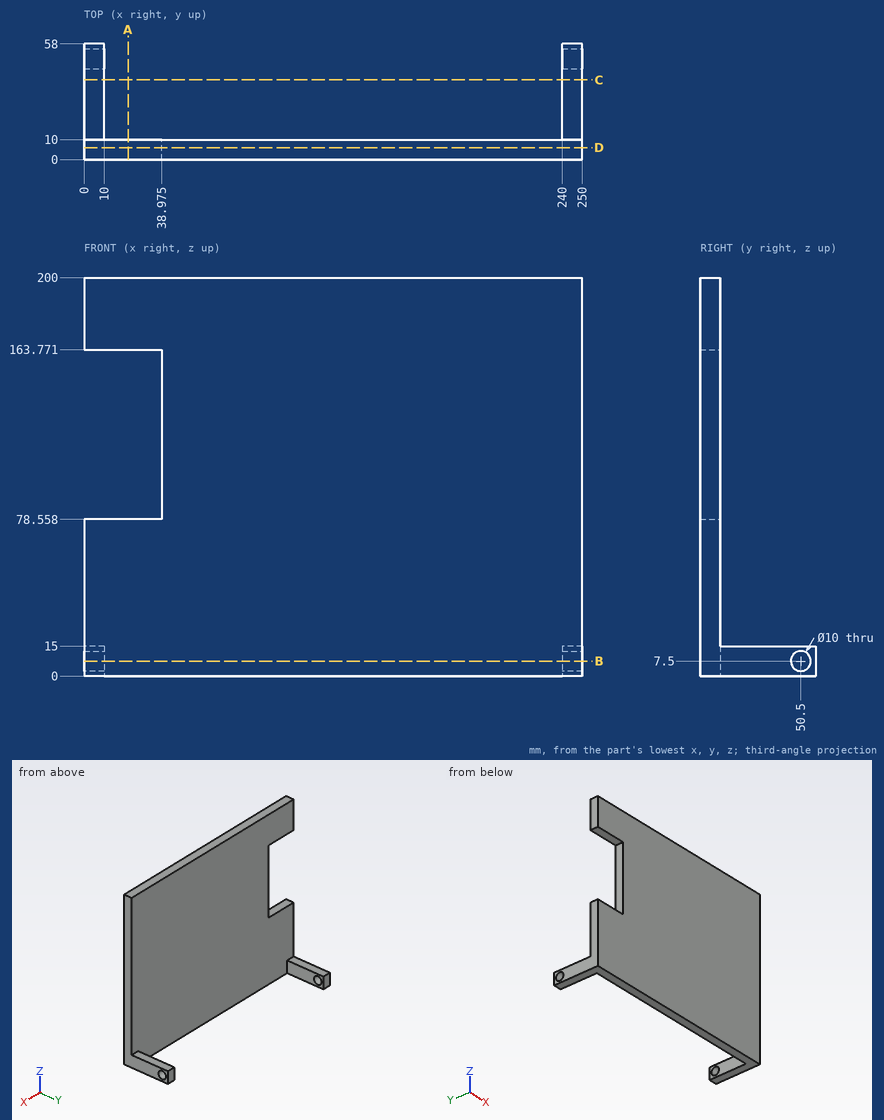
Can you work these out from the drawing? Everything is in mm from the part's minimum corner. Give positions to 0.01 mm unless a question says otherwise; leave off trailing zeros. Loops run counter-clockwise (first coordinate to the right, second up) from the corner with the lowest first, then second, coordinate; pieces in that order, holes last. Notation, with made-up numbers: M 10,80 L 23,80 A11 cw 23,98 Z; hole C 15.25,40 d5. An arc over 180 degrees is marked long. Put each result on its own line as item: value. Start each with the question number.
(1) I need wall thicknesses on line 1 along Z through (x, y) = (6, 50) (1 decimal); line 2 along Y through (x, z) = (246, 7.5); line 3 along Y through (x, z) = (205, 101). Which ranges of each line are inside material? Lowest first, please. Write a range as [from, to].
(2) I want a section at A-A on x = 22. Please give me the cut outline in (y, z), then the cut area to 3 significant figures.
(3) I want a section at D-D on y = 6. Please give me the cut outline in (x, z) (1 decimal).
(4) I want a section at B-B on z = 7.5. Please give me the cut outline in (x, y), then the cut area to 3 significant figures.
(5) Will these pins go through, and if not, where does the flat tip stop? pin 1 Ø8 at (x, z) = (101, 127) entering from +Y; pin 2 Ø3 at (x, y) = (6.5, 43) entering from +Z; pin 3 Ø8 at (y, z) = (2.5, 116) entering from -X (3 decimals).
(6) I want a section at C-C on y = 40. Please give me the cut outline in (x, z), then the cut area to 3 significant figures.
Answer block:
1. line 1: [0, 2.5], [12.5, 15]
1. line 2: [0, 45.5], [55.5, 58]
1. line 3: [0, 10]
2. outline: M 0,0 L 10,0 L 10,78.56 L 0,78.56 Z; M 0,163.77 L 10,163.77 L 10,200 L 0,200 Z
2. area: 1,150 mm^2
3. outline: M 0,0 L 250,0 L 250,200 L 0,200 L 0,163.8 L 39,163.8 L 39,78.6 L 0,78.6 Z
4. outline: M 0,0 L 250,0 L 250,45.5 L 240,45.5 L 240,10 L 10,10 L 10,45.5 L 0,45.5 Z; M 0,55.5 L 10,55.5 L 10,58 L 0,58 Z; M 240,55.5 L 250,55.5 L 250,58 L 240,58 Z
4. area: 3,260 mm^2
5. pin 1: y = 10
5. pin 2: z = 15
5. pin 3: x = 38.975
6. outline: M 0,0 L 10,0 L 10,15 L 0,15 Z; M 240,0 L 250,0 L 250,15 L 240,15 Z
6. area: 300 mm^2
